from build123d import *

# Parameters (mm, degrees)
F1_DEPTH = 300
F2_R     = 1
F3_R     = 2.38125
F4_R     = 2.5
F5_DEPTH = 25
F6_SIZE  = 0.5


with BuildPart() as f1:
    # F0 (on Right) → F1 (new body, symmetric)
    with BuildSketch(Plane.YZ):
        Polygon((0, 25.4), (0, 0), (25.4, 0), (25.4, 4.7625), (4.7625, 4.7625), (4.7625, 25.4), align=None)
    extrude(amount=F1_DEPTH, both=True)

    # F2
    f2_edges = [f1.edges().sort_by_distance(p)[0] for p in [
        (0, 0, 25.4),
        (0, 4.7625, 25.4),
        (0, 0, 0),
        (0, 25.4, 4.7625),
        (0, 25.4, 0),
    ]]
    fillet(f2_edges, radius=F2_R)

    # F3
    f3_edges = [f1.edges().sort_by_distance(p)[0] for p in [
        (0, 4.7625, 4.7625),
    ]]
    fillet(f3_edges, radius=F3_R)

    # F4 (on face) → F5 (cut)
    with BuildSketch(Plane.XY.offset(4.7625)):
        with Locations((0, 15)):
            Circle(F4_R)
    extrude(amount=-F5_DEPTH, mode=Mode.SUBTRACT)

    # F6
    f6_edges = [f1.edges().sort_by_distance(p)[0] for p in [
        (-2.5, 15, 4.7625),
        (2.5, 15, 2.38125),
        (-2.5, 15, 0),
    ]]
    chamfer(f6_edges, length=F6_SIZE)


solid = f1.part
The model under review builds one solid part; all positions refer to its coordinate system, in mm. A direction names the side the tool comes from. Round coordinates to 2 decimals unless told otherwise and drop trailing zeros. Loops run counter-clockwise (first coordinate to the right, second up) from the corner with the lowest first, then second, coordinate; pieces in that order, holes last. Notation, with made-up numbers: (78, -16.5) - (115, -16.5) arc R31 ccw to (115, 8.5) - close; hole circle Ø4 at (-32.75, 48.25). An arc over 180 degrees is marked (long way). Use CSV: the item, a comma, the result in double quotes.
(1) Machinability: for faces 1 (the flat face through (300, 4, 7)), 2 (the flat face through (4, 16, 4.762)), which of the approach directions +Z, -Z, +X, -X, +Y, -Y give a long, thin tool a straight path to every point of the face, cutting with its end or side? Answer none if there is none.
Working result:
face 1,"+Z, -Z, +X, +Y, -Y"
face 2,"+Z, +X, -X, +Y"
(2) Take a section at B-B, the plane z = 12.5. Give the boundary of the cut face in (x, y).
Working result:
outline,"(-300, 0) - (300, 0) - (300, 4.76) - (-300, 4.76) - close"
(3) Take a section at A-A, the plane x = -21. Give the boundary of the cut face in (y, z), plus the area to 3 significant figures.
Working result:
outline,"(0, 1) arc R1 ccw to (1, 0) - (24.4, 0) arc R1 ccw to (25.4, 1) - (25.4, 3.76) arc R1 ccw to (24.4, 4.76) - (7.14, 4.76) arc R2.38 cw to (4.76, 7.14) - (4.76, 24.4) arc R1 ccw to (3.76, 25.4) - (1, 25.4) arc R1 ccw to (0, 24.4) - close"
area,"219 mm^2"
(4) For line 1 (Y direction, x = 0, z = 1.5); line 2 (Z direction, x = -264.5, y = 14), list the stretches that pass through material, from the lowest coordinate up.
Working result:
line 1,"y = 0 to 12.5, 17.5 to 25.4"
line 2,"z = 0 to 4.76"
(5) Clearance check with flat-ended pins moving along their axes: P1, Ø5, axis at x = -87, y = 14, coming from the +Z side; P2, Ø14, axis at x = -39.5, z = 16.5, coming from the +Y side; P3, Ø8, axis at x = 231.5, y = 10.5, coming from the +Z side. State where each tip first meets the part, or that it passes through.
Working result:
P1,"stops at z = 4.76"
P2,"stops at y = 4.76"
P3,"stops at z = 4.85"
